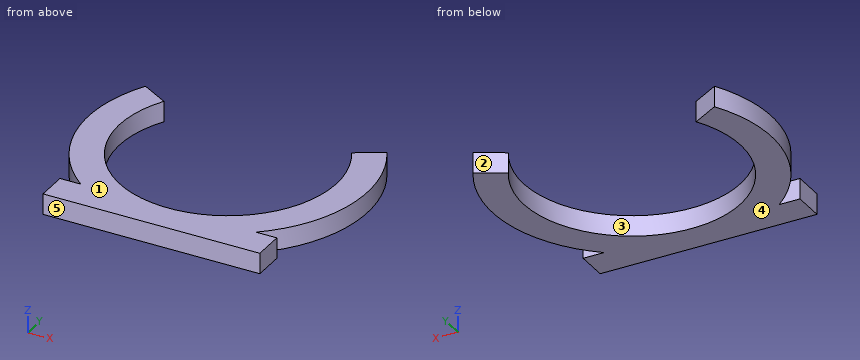
from build123d import *

# Parameters (mm, degrees)
BOSS_EXTRUDE1_DEPTH = 2


with BuildPart() as part:
    # Sketch1 → Boss-Extrude1 (new body)
    with BuildSketch(Plane.XY):
        with BuildLine():
            Line((-9.09326674, 5.25), (-11.691342951, 6.75))
            ThreePointArc((-11.691342951, 6.75), (-13.272703843, -2.466846714), (-8.485281374, -10.5))
            Line((-8.485281374, -10.5), (-10.5, -10.5))
            Line((-10.5, -10.5), (-10.5, -13.5))
            Line((-10.5, -13.5), (10.5, -13.5))
            Line((10.5, -13.5), (10.5, -10.5))
            Line((10.5, -10.5), (8.485281374, -10.5))
            ThreePointArc((8.485281374, -10.5), (13.272703843, -2.466846714), (11.691342951, 6.75))
            Line((11.691342951, 6.75), (9.09326674, 5.25))
            ThreePointArc((9.09326674, 5.25), (0, -10.5), (-9.09326674, 5.25))
        make_face()
    extrude(amount=BOSS_EXTRUDE1_DEPTH)


solid = part.part
Here's how the part is built. I have some questions about the finished solid (model axes, mm). Face numbers are marked on the shaded views. A direction names the side the tool comes from. Round coordinates to 2 decimals unless told otherwise and drop trailing zeros. Write each loop counter-clockwise with the first axis right and the second up, starting at its lowest first coordinate (ties: lowest second). Pieces come first, ordered by that corner, then holes.
1. Suppose I cut it at D-D (y = -6). List the corners of the cut face in (x, z) for me.
2. Suppose I cut it at B-B (z = 1.4). List the corners of the cut face in (x, y) for me, and give its area (3 significant figures).
3. For the marked faces 1 and 2, which set-ups out of +Z, -Z, +X, -X, +Y, -Y let a thin tool reach every point of the face, with its end or its side?
4. Suppose I cut it at A-A (y = 0). List the corners of the cut face in (x, z) for me.
5. Suppose I cut it at C-C (x = 0). List the corners of the cut face in (y, z) for me, and give its area (3 significant figures).
6. If we mould it in two halves opening along Y, with no side actions, what happens to the marked faces 3, 4 and 5? For each: released by +Y, released by -Y, zero draft, split by the parting line, or undercut.
7. Will these pins go through, and if not, where does the flat tip stop? pin 1 Ø0.6 at (y, z) = (-11.5, 1) entering from -X; pin 2 Ø1 at (x, z) = (-10, 0.5) entering from +Y; pin 3 Ø0.6 at (x, z) = (10, 0.5) entering from +Y.
8. I need wall thicknesses on L1, parallel to X at y = 0, z = 0.6; L2, parallel to Y at x = 0, z = 0.4; L3, parallel to X at y = -5.25, z = 1.75. Which ranges of each line are inside material? Lowest first, please.
Answer sheet:
1. outline: (-12.09, 0) - (-8.62, 0) - (-8.62, 2) - (-12.09, 2) - close; (8.62, 0) - (12.09, 0) - (12.09, 2) - (8.62, 2) - close
2. outline: (-11.69, 6.75) arc R13.5 ccw to (-8.49, -10.5) - (-10.5, -10.5) - (-10.5, -13.5) - (10.5, -13.5) - (10.5, -10.5) - (8.49, -10.5) arc R13.5 ccw to (11.69, 6.75) - (9.09, 5.25) arc R10.5 cw (long way) to (-9.09, 5.25) - close
2. area: 179 mm2
3. face 1: +Z, +X, -X, +Y, -Y
3. face 2: +Z, -Z, +Y
4. outline: (-13.5, 0) - (-10.5, 0) - (-10.5, 2) - (-13.5, 2) - close; (10.5, 0) - (13.5, 0) - (13.5, 2) - (10.5, 2) - close
5. outline: (-13.5, 0) - (-10.5, 0) - (-10.5, 2) - (-13.5, 2) - close
5. area: 6.00 mm2
6. face 3: undercut
6. face 4: zero draft
6. face 5: released by -Y
7. pin 1: stops at x = -10.5
7. pin 2: stops at y = 6.06
7. pin 3: stops at y = 5.95
8. L1: x = -13.5 to -10.5, 10.5 to 13.5
8. L2: y = -13.5 to -10.5
8. L3: x = -12.44 to -9.09, 9.09 to 12.44
